Geometry check sheet. Reference: the model listing, model coordinates, mm. A direction names the side the tool comes from. Coordinates: 2 decimals unless noted, no trailing zeros. Write each loop counter-clockwise with the first axis right and the second up, starting at its lowest first coordinate (ties: lowest second). Pieces come first, ordered by that corner, then holes. Notation, with made-up numbers: M 5,58.5 L 33,58.5 A10 ccw 33,71.5 Z; hole C -38.75,-2 d4. An arc over 180 degrees is marked long. Put each result on its own line as item: value. Start each with the question number.
1) Cross-section at C-C on z = -9. Record the cut outline in (x, y).
2) Cross-section at B-B on y = 20. Record the cut outline in (x, z).
3) Scan lines: line 1 along X through (y, z) = (6.75, 22); line 2 along X through (y, z) = (11.75, 21.5); line 3 along Z through (x, y) = (67, 9). Record each from-to range of solid material in increasing order.
4) Mould release check, pull along Z, two halves, no side actions. Record for faces 1 (the flat face through (10, 10.6, -7)), 2 (the cylindrical face through (-70.72, 12.32, -21.97)), 3 (the flat face through (-3, 6, 33.5)): released by +Z, released by -Z, zero draft, split by the parting line, or undercut.
5) Cross-section at D-D on x = -8.2. Record the cut outline in (y, z), plus the area to 3 significant figures.
6) Gauge pin test, flat ends, axial feed: pin 1 (3 mm diameter, centred on y = 13.5, z = 31.5, fed in from -X); pin 2 (0.9 mm diameter, centred on x = -78, z = 32, fed in from +Y); pin 3 (1.6 mm diameter, centred on y = 10, z = 12.5, fed in from -X). Record the tip position at first contact, or that the pin passes through.
7) Set-up check for faces 4 (the flat face through (-40.2, 13, 0)), 5 (the flat face through (-63.2, 20, 0)), 6 (the flat face through (5, 9.1, 16)), 7 (the flat face through (-75, 18, -30.5)): record each of +Z, -Z, +X, -X, +Y, -Y from which the full face is reachable in a straight line by a thin tool's end or side.
8) Cross-section at A-A on x = 74.1. Record the cut outline in (y, z), plus the area to 3 significant figures.
from build123d import *

# Parameters (mm, degrees)
SKETCH1_W           = 195
SKETCH1_H           = 67
BOSS_EXTRUDE1_DEPTH = 25
CUT_EXTRUDE1_DEPTH  = 107.082515053
CUT_EXTRUDE2_DEPTH  = 121.914225797
CUT_EXTRUDE3_START  = -13
SKETCH4_W           = 3.612655346
SKETCH4_H           = 3
CUT_EXTRUDE3_DEPTH  = 13
SKETCH6_R           = 2.5
CUT_EXTRUDE4_DEPTH  = 107.082515053
SKETCH7_W           = 37
SKETCH7_H           = 35
CUT_EXTRUDE5_DEPTH  = 1.5
CUT_EXTRUDE6_DEPTH  = 18.5


with BuildPart() as part:
    # Sketch1 → Boss-Extrude1 (new body)
    with BuildSketch(Plane(origin=(0, 0, 0), x_dir=(1, 0, 0), z_dir=(0, 1, 0))):
        Rectangle(SKETCH1_W, SKETCH1_H)
    extrude(amount=BOSS_EXTRUDE1_DEPTH)

    # Sketch2 → Cut-Extrude1 (cut, through all)
    with BuildSketch(Plane.XZ):
        with BuildLine():
            Line((97.5, -3.219751644), (97.5, 33.5))
            Line((97.5, 33.5), (88.5, 33.5))
            ThreePointArc((88.5, 33.5), (95.217186872, 15.683556008), (97.5, -3.219751644))
        make_face()
        with BuildLine():
            Line((97.5, -33.5), (97.5, -3.219751644))
            ThreePointArc((97.5, -3.219751644), (95.985558513, -18.65423771), (91.5, -33.5))
            Line((91.5, -33.5), (97.5, -33.5))
        make_face()
        with BuildLine():
            ThreePointArc((-88, -33.5), (-95.08607052, -15.861694529), (-97.5, 2.992884749))
            Line((-97.5, 2.992884749), (-97.5, -33.5))
            Line((-97.5, -33.5), (-88, -33.5))
        make_face()
        with BuildLine():
            ThreePointArc((-97.5, 2.992884749), (-95.856964648, 18.588830376), (-91, 33.5))
            Line((-91, 33.5), (-97.5, 33.5))
            Line((-97.5, 33.5), (-97.5, 2.992884749))
        make_face()
    extrude(amount=-CUT_EXTRUDE1_DEPTH, mode=Mode.SUBTRACT)

    # Sketch3 → Cut-Extrude2 (cut, through all)
    with BuildSketch(Plane(origin=(0, 0, 33.5), x_dir=(-1, 0, 0), z_dir=(0, 0, -1))):
        Polygon((63.2, 25), (63.2, 14.6), (40.2, 14.6), (40.2, 10.6), (-61.8, 10.6), (-61.8, 14.6), (-97.5, 14.6), (-97.5, 25), align=None)
    extrude(amount=CUT_EXTRUDE2_DEPTH, mode=Mode.SUBTRACT)

    # Sketch4 → Cut-Extrude3 (cut)
    with BuildSketch(Plane(origin=(0, 25, 0), x_dir=(1, 0, 0), z_dir=(0, 1, 0)).offset(CUT_EXTRUDE3_START)):
        with BuildLine():
            Line((-63.2, 30.5), (-63.2, 33.5))
            Line((-63.2, 33.5), (-88, 33.5))
            ThreePointArc((-88, 33.5), (-88.810680862, 32.008999469), (-89.587344654, 30.5))
            Line((-89.587344654, 30.5), (-63.2, 30.5))
        make_face()
        with Locations((-61.393672327, 32)):
            Rectangle(SKETCH4_W, SKETCH4_H)
        with BuildLine():
            Line((-63.2, -33.5), (-63.2, -30.5))
            Line((-63.2, -30.5), (-92.261692194, -30.5))
            ThreePointArc((-92.261692194, -30.5), (-91.647155152, -32.006859002), (-91, -33.5))
            Line((-91, -33.5), (-63.2, -33.5))
        make_face()
        with Locations((-61.393672327, -32)):
            Rectangle(SKETCH4_W, SKETCH4_H)
    extrude(amount=CUT_EXTRUDE3_DEPTH, mode=Mode.SUBTRACT)

    # Sketch6 → Cut-Extrude4 (cut, through all)
    with BuildSketch(Plane.XZ):
        with Locations(Location((-28.1, -9, 0), (0, 0, 270))):
            Circle(SKETCH6_R)
        with Locations(Location((-8.2, -8.3, 0), (0, 0, 270))):
            Circle(SKETCH6_R)
        with Locations(Location((-18.7, 8.7, 0), (0, 0, 270))):
            Circle(SKETCH6_R)
        with Locations(Location((-76.2, 22, 0), (0, 0, 270))):
            Circle(SKETCH6_R)
        with Locations(Location((-78.2, 0.1, 0), (0, 0, 270))):
            Circle(SKETCH6_R)
        with Locations(Location((-73.2, -22.3, 0), (0, 0, 270))):
            Circle(SKETCH6_R)
        with Locations(Location((65.3, -20, 0), (0, 0, 270))):
            Circle(SKETCH6_R)
        with Locations(Location((74.1, -1.7, 0), (0, 0, 270))):
            Circle(SKETCH6_R)
        with Locations(Location((68.3, 21.5, 0), (0, 0, 270))):
            Circle(SKETCH6_R)
    extrude(amount=-CUT_EXTRUDE4_DEPTH, mode=Mode.SUBTRACT)

    # Sketch7 → Cut-Extrude5 (cut)
    with BuildSketch(Plane(origin=(0, 10.6, 0), x_dir=(1, 0, 0), z_dir=(0, 1, 0))):
        with Locations((5.3, -16)):
            Rectangle(SKETCH7_W, SKETCH7_H)
    extrude(amount=-CUT_EXTRUDE5_DEPTH, mode=Mode.SUBTRACT)

    # Sketch8 → Cut-Extrude6 (cut)
    with BuildSketch(Plane(origin=(0, 25, 0), x_dir=(1, 0, 0), z_dir=(0, 1, 0))):
        with BuildLine():
            Line((37.096152423, 33.5), (31.9, 33.5))
            Line((31.9, 33.5), (31.9, 30.5))
            ThreePointArc((31.9, 30.5), (34.9, 31.303847577), (37.096152423, 33.5))
        make_face()
        with BuildLine():
            Line((31.9, 33.5), (26.703847577, 33.5))
            ThreePointArc((26.703847577, 33.5), (28.9, 31.303847577), (31.9, 30.5))
            Line((31.9, 30.5), (31.9, 33.5))
        make_face()
    extrude(amount=-CUT_EXTRUDE6_DEPTH, mode=Mode.SUBTRACT)


solid = part.part
Answer key:
1. outline: M -96.53,0 L -30.6,0 L -30.6,10.6 L -40.2,10.6 L -40.2,14.6 L -63.2,14.6 L -63.2,25 L -96.53,25 Z; M -25.6,0 L -10.6,0 L -10.6,10.6 L -25.6,10.6 Z; M -5.8,0 L 97.29,0 L 97.29,14.6 L 61.8,14.6 L 61.8,10.6 L -5.8,10.6 Z
2. outline: M -92.26,30.5 A74.84 ccw -89.59,-30.5 L -63.2,-30.5 L -63.2,30.5 Z; hole C -78.2,0.1 d5; hole C -76.2,22 d5; hole C -73.2,-22.3 d5
3. line 1: x = -95.05 to -78.7, -73.7 to 65.85, 70.75 to 93.39
3. line 2: x = -95.18 to -78.65, -73.75 to -40.2, 61.8 to 65.8, 70.8 to 93.55
3. line 3: z = -33.5 to -21.83, -18.17 to 19.36, 23.64 to 33.5
4. face 1: zero draft
4. face 2: undercut
4. face 3: released by +Z
5. outline: M 0,-33.5 L 10.6,-33.5 L 10.6,-10.8 L 0,-10.8 Z; M 0,-5.8 L 10.6,-5.8 L 10.6,-1.5 L 9.1,-1.5 L 9.1,33.5 L 0,33.5 Z
5. area: 605 mm²
6. pin 1: stops at x = -92.46
6. pin 2: stops at y = 12
6. pin 3: stops at x = -96.99
7. face 4: +Z, -Z, +Y
7. face 5: +Z, -Z, +X, +Y
7. face 6: +Z, +Y
7. face 7: -Z, -X, +Y
8. outline: M 0,-33.5 L 14.6,-33.5 L 14.6,-4.2 L 0,-4.2 Z; M 0,0.8 L 14.6,0.8 L 14.6,33.5 L 0,33.5 Z
8. area: 905 mm²
